Build history of the part. All positions in model axes, mm. Round coordinates to 2 decimals unless told otherwise and drop trailing zeros. Order: outer loops, then holes, each group sorted by start corner. A loop starts at its lowest first (then second) coordinate and runs counter-clockwise, first axis right, second up. Notation, with made-up numbers: (30.25, 37) -> (62.25, 37) arc R10 cw to (62.25, 47) -> close; hole circle Ø2 at (23, 84). An arc over 180 degrees is marked (long way). Write item = value, one per line.
from build123d import *

# Parameters (mm, degrees)
BOSS_EXTRU_1_DEPTH      = 254.666666667
ESQUISSE4_R             = 51.382798763
ESQUISSE4_R_2           = 27.5
ENL_V_MAT_EXTRU_1_DEPTH = 265.098930571
ESQUISSE5_R             = 10
ESQUISSE5_R_2           = 3
ESQUISSE5_W             = 1.7
ESQUISSE5_H             = 10
ENL_V_MAT_EXTRU_2_DEPTH = 258.285428534


with BuildPart() as part:
    # Esquisse1 → Boss.-Extru.1 (new body)
    with BuildSketch(Plane.XY):
        with BuildLine():
            Line((-17.5, -48.310889132), (-17.5, -47.310889132))
            ThreePointArc((-17.5, -47.310889132), (-9, -15.588457268), (-32.222431864, -38.810889132))
            Line((-32.222431864, -38.810889132), (-33.088457268, -39.310889132))
            ThreePointArc((-33.088457268, -39.310889132), (-35.314540075, -27.733649929), (-29.89862988, -17.26198201))
            ThreePointArc((-29.89862988, -17.26198201), (-41.675315415, -16.716463864), (-50.588457268, -9))
            Line((-50.588457268, -9), (-49.722431864, -8.5))
            ThreePointArc((-49.722431864, -8.5), (-18, 0), (-49.722431864, 8.5))
            Line((-49.722431864, 8.5), (-50.588457268, 9))
            ThreePointArc((-50.588457268, 9), (-41.675315415, 16.716463864), (-29.89862988, 17.26198201))
            ThreePointArc((-29.89862988, 17.26198201), (-35.314540075, 27.733649929), (-33.088457268, 39.310889132))
            Line((-33.088457268, 39.310889132), (-32.222431864, 38.810889132))
            ThreePointArc((-32.222431864, 38.810889132), (-9, 15.588457268), (-17.5, 47.310889132))
            Line((-17.5, 47.310889132), (-17.5, 48.310889132))
            ThreePointArc((-17.5, 48.310889132), (-6.36077534, 44.450113792), (0, 34.523964019))
            ThreePointArc((0, 34.523964019), (6.36077534, 44.450113792), (17.5, 48.310889132))
            Line((17.5, 48.310889132), (17.5, 47.310889132))
            ThreePointArc((17.5, 47.310889132), (9, 15.588457268), (32.222431864, 38.810889132))
            Line((32.222431864, 38.810889132), (33.088457268, 39.310889132))
            ThreePointArc((33.088457268, 39.310889132), (35.314540075, 27.733649929), (29.89862988, 17.26198201))
            ThreePointArc((29.89862988, 17.26198201), (41.675315415, 16.716463864), (50.588457268, 9))
            Line((50.588457268, 9), (49.722431864, 8.5))
            ThreePointArc((49.722431864, 8.5), (18, 0), (49.722431864, -8.5))
            Line((49.722431864, -8.5), (50.588457268, -9))
            ThreePointArc((50.588457268, -9), (41.675315415, -16.716463864), (29.89862988, -17.26198201))
            ThreePointArc((29.89862988, -17.26198201), (35.314540075, -27.733649929), (33.088457268, -39.310889132))
            Line((33.088457268, -39.310889132), (32.222431864, -38.810889132))
            ThreePointArc((32.222431864, -38.810889132), (9, -15.588457268), (17.5, -47.310889132))
            Line((17.5, -47.310889132), (17.5, -48.310889132))
            ThreePointArc((17.5, -48.310889132), (6.36077534, -44.450113792), (0, -34.523964019))
            ThreePointArc((0, -34.523964019), (-6.36077534, -44.450113792), (-17.5, -48.310889132))
        make_face()
    extrude(amount=BOSS_EXTRU_1_DEPTH)

    # Esquisse4 → Enlèv. mat.-Extru.1 (cut, through all)
    with BuildSketch(Plane.XY.offset(254.666666667)):
        Circle(ESQUISSE4_R)
        Circle(ESQUISSE4_R_2, mode=Mode.SUBTRACT)
    extrude(amount=-ENL_V_MAT_EXTRU_1_DEPTH, mode=Mode.SUBTRACT)

    # Esquisse5 → Enlèv. mat.-Extru.2 (cut, through all)
    with BuildSketch(Plane.XY.offset(254.666666667)):
        Circle(ESQUISSE5_R)
        with Locations((0, 15)):
            Circle(ESQUISSE5_R_2)
        with Locations((12.990381057, 7.5)):
            Circle(ESQUISSE5_R_2)
        with Locations((12.990381057, -7.5)):
            Circle(ESQUISSE5_R_2)
        with Locations((0, -15)):
            Circle(ESQUISSE5_R_2)
        Polygon((13.706088614, -13.739641853), (5.045834576, -18.739641853), (4.195834576, -17.267398667), (12.856088614, -12.267398667), align=None)
        Polygon((17.051923191, 5), (18.751923191, 5), (18.751923191, -5), (17.051923191, -5), (17.051923191, -1.5), (13.051923191, -1.5), (13.051923191, 1.5), (17.051923191, 1.5), align=None)
        Polygon((-5.045834576, -18.739641853), (-13.706088614, -13.739641853), (-12.856088614, -12.267398667), (-4.195834576, -17.267398667), align=None)
        with Locations((-17.901923191, 0)):
            Rectangle(ESQUISSE5_W, ESQUISSE5_H)
        Polygon((-13.706088614, 13.739641853), (-5.045834576, 18.739641853), (-4.195834576, 17.267398667), (-12.856088614, 12.267398667), align=None)
        Polygon((5.045834576, 18.739641853), (13.706088614, 13.739641853), (12.856088614, 12.267398667), (4.195834576, 17.267398667), align=None)
    extrude(amount=-ENL_V_MAT_EXTRU_2_DEPTH, mode=Mode.SUBTRACT)


solid = part.part
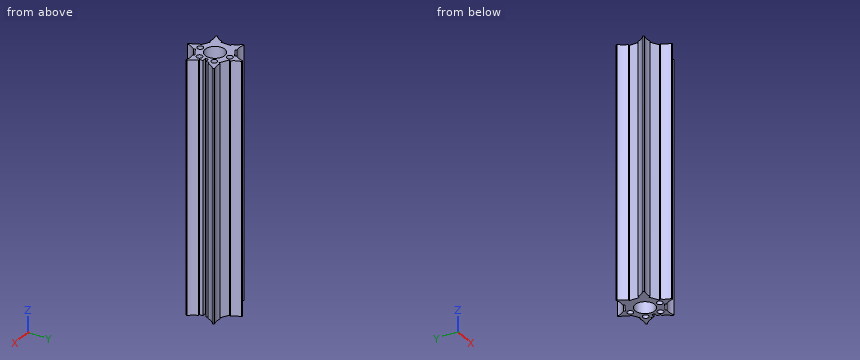
Q1. Cut at A-A, the plane x = 21. List the corners of the cut face in (y, z), and give its area (3 significant figures).
Check values:
outline = (-13.68, 0) -> (-9.64, 0) -> (-9.64, 254.67) -> (-13.68, 254.67) -> close; (9.64, 0) -> (13.68, 0) -> (13.68, 254.67) -> (9.64, 254.67) -> close
area = 2,050 mm²
Q2. Cut at C-C, the plane z = 127. Give the number of separate pieces and of enclosed holes in the cut face, and give its area (3 significant figures).
Check values:
separate_pieces = 1
enclosed_holes = 5
area = 836 mm²
Q3. Flat gauge pins, fed straight in: pin 1 (0.5 mm diameter, centred on x = 18, z = 179, fed in from -Y); pin 2 (6 mm diameter, centred on x = 6.5, z = 60, fed in from -Y); pin 3 (10 mm diameter, centred on x = -13, z = 82.5, fed in from +Y). Where does each tip first touch, or does it go through?
Check values:
pin_1 = -13.33
pin_2 = -20.67
pin_3 = 15.07
Q4. Cut at B-B, the plane y = -7.5. List the corners of the cut face in (x, z), and give its area (3 significant figures).
Check values:
outline = (-19.74, 0) -> (-6.61, 0) -> (-6.61, 254.67) -> (-19.74, 254.67) -> close; (6.61, 0) -> (9.99, 0) -> (9.99, 254.67) -> (6.61, 254.67) -> close; (15.99, 0) -> (19.74, 0) -> (19.74, 254.67) -> (15.99, 254.67) -> close
area = 5,160 mm²
Q5. Probe probe 1 along Y at (x, z) = (0, 178.5); probe 2 along Y at (x, z) = (10.5, 142.5); probe 3 along Y at (x, z) = (12, 157). List the from-to ranges inside material, lowest first.
Check values:
probe_1 = -27.5 to -18, -12 to -10, 10 to 12, 18 to 27.5
probe_2 = -13.63 to -9.17, -5.83 to 5.83, 9.17 to 13.63
probe_3 = -12.76 to -10.33, -4.67 to 4.67, 10.33 to 12.76
